The listing builds one solid part. Answer for the finished solid, in the listing's coordinates (mm). A direction names the side the tool comes from. Coordinates: 2 decimals unless noted, no trailing zeros. Order: outer loops, then holes, each group sorted by start corner. A loop starts at its lowest first (then second) coordinate and runs counter-clockwise, first axis right, second up.
```python
from build123d import *

# Parameters (mm, degrees)
F3_R           = 10
F4_R           = 12
F6_D           = 3
F6_CBORE_D     = 5.75
F6_CBORE_DEPTH = 1


with BuildPart() as f2:
    # F2: sweep along a path in F1
    with BuildLine(Plane.XY) as f2_path:
        Line((-6.2, 0), (-6.2, 80))
        Line((-6.2, 80), (73.8, 80))
    # F0 (on Front) → F2 (sweep)
    with BuildSketch(Plane.XZ):
        Polygon((-6.2, -3), (-6.2, -1), (-2, -1), (-2, 0), (0, 0), (0, 1.25), (-13.2, 1.25), (-13.2, -3), align=None)
    sweep(path=f2_path.line, transition=Transition.RIGHT)

    # F3
    f3_edges = [f2.edges().sort_by_distance(p)[0] for p in [
        (-13.2, 0, -0.875),
        (73.8, 87, -0.875),
    ]]
    fillet(f3_edges, radius=F3_R)

    # F4
    f4_edges = [f2.edges().sort_by_distance(p)[0] for p in [
        (-13.2, 87, -0.875),
    ]]
    fillet(f4_edges, radius=F4_R)

    # F6 (through all)
    with Locations(Plane.XY.offset(1.25)):
        with Locations((-3.65, 77.45)):
            CounterBoreHole(F6_D / 2, F6_CBORE_D / 2, F6_CBORE_DEPTH)


solid = f2.part
```
(1) The mould has two halves that part along X. Classify faces 1 (the face through (70.79, 84.15, -0.9)), 2 (the face through (-4.456, 78.715, -0.384)), 3 (the face through (19, 75, 0)): released by +X, released by -X, zero draft, split by the parting line, or undercut.
(2) Consider line 1 (Z direction, x = -2.5, y = 71); line 2 (X direction, y = 77.45, z = -0.25); line 3 (Y direction, x = -3.65, z = 1) (3 decimals). Determine where each line is inside the solid, lowest interval first.
(3) Find section C-C (x = 42.5). Write down the section's boundary in (y, z).
(4) Find section B-B (z = -2.1). Write down the section's boundary in (x, y), and give its area (3 significant figures).
(5) Find section A-A (y = 58.5). Write down the section's boundary in (x, z), and give its area (3 significant figures).
(6) For faces 4 (the face through (-5, 58, -1)), 5 (the face through (-2, 76, 0.25)), 6 (the face through (-1.9, 0, 0.4)), determine the directions among +Z, -Z, +X, -X, +Y, -Y from which every point of the face is accessible in a straight line to the end or side of a thin tool.
(7) Each of these flat-tipped pins is pushed along its axis until it touches: pin 1 Ø2 at (y, z) = (46, -1.5) entering from +X; pin 2 Ø0.6 at (x, z) = (49.5, 0.5) entering from -Y; pin 3 Ø10 at (x, y) = (4, 17.5) entering from -Z; pin 4 Ø6.5 at (x, y) = (-3.65, 77.45) entering from -Z. Where does it stop, or does it pass through?
Findings below:
1. face 1: released by +X
1. face 2: undercut
1. face 3: zero draft
2. line 1: z = -1 to 1.25
2. line 2: x = -12.95 to -5.15, -2.15 to 73.79
2. line 3: y = 0.01 to 74.575, 80.325 to 86.747
3. outline: (73.8, 0) - (75.8, 0) - (75.8, -1) - (80, -1) - (80, -3) - (87, -3) - (87, 1.25) - (73.8, 1.25) - close
4. outline: (-13.2, 10) arc R10 ccw to (-6.2, 0.46) - (-6.2, 80) - (73.34, 80) arc R10 ccw to (63.8, 87) - (-1.2, 87) arc R12 ccw to (-13.2, 75) - close
4. area: 1,100 mm2
5. outline: (-13.2, -3) - (-6.2, -3) - (-6.2, -1) - (-2, -1) - (-2, 0) - (0, 0) - (0, 1.25) - (-13.2, 1.25) - close
5. area: 41.7 mm2
6. face 4: -Z, +X, -Y
6. face 5: +Z
6. face 6: +Z, -Z, +X, -X, -Y
7. pin 1: stops at x = -2
7. pin 2: stops at y = 73.8
7. pin 3: stops at z = 0
7. pin 4: stops at z = -3
